Here's the drawing with two shaded views (mm, measured from the low corner). I have some questions. A direction names the side the tool comes from. Round coordinates to 2 decimals unless told otherwise and drop trailing zeros. Loops run counter-clockwise (first coordinate to the right, second up) from the corner with the lowest first, then second, coordinate; pieces in that order, holes last.
(1) If I drill on line 1 along Z through (x, y) = (16, 16); line 2 along X through (y, z) = (17.5, 56); line 3 along Z through (x, y) = (104, 17.75), over which ranges is the centre line in solid material (lowest first)?
(2) I want a section at C-C on z = 72. Write out the boundary of the cut face in (x, y).
(3) I want a section at A-A on y = 8. Write out the boundary of the cut face in (x, z) (1 decimal), plus the area to 3 significant figures.
(4) Will these pins go through, and if not, where does the flat tip stop? pin 1 Ø4 at (x, y) = (58, 11) entering from +Z; pin 2 Ø0.9 at (x, y) = (81.5, 17) entering from +Z; pin 3 Ø3 at (x, y) = (128, 16) entering from +Z.
(5) I want a section at B-B on x = 113. Write out the boundary of the cut face in (y, z).
(6) Which directions (+Z, -Z, +X, -X, +Y, -Y) give clear straight access to the entire face, cutting with the end or side of a thin tool? Please do the marked faces 1, 2 and 3.
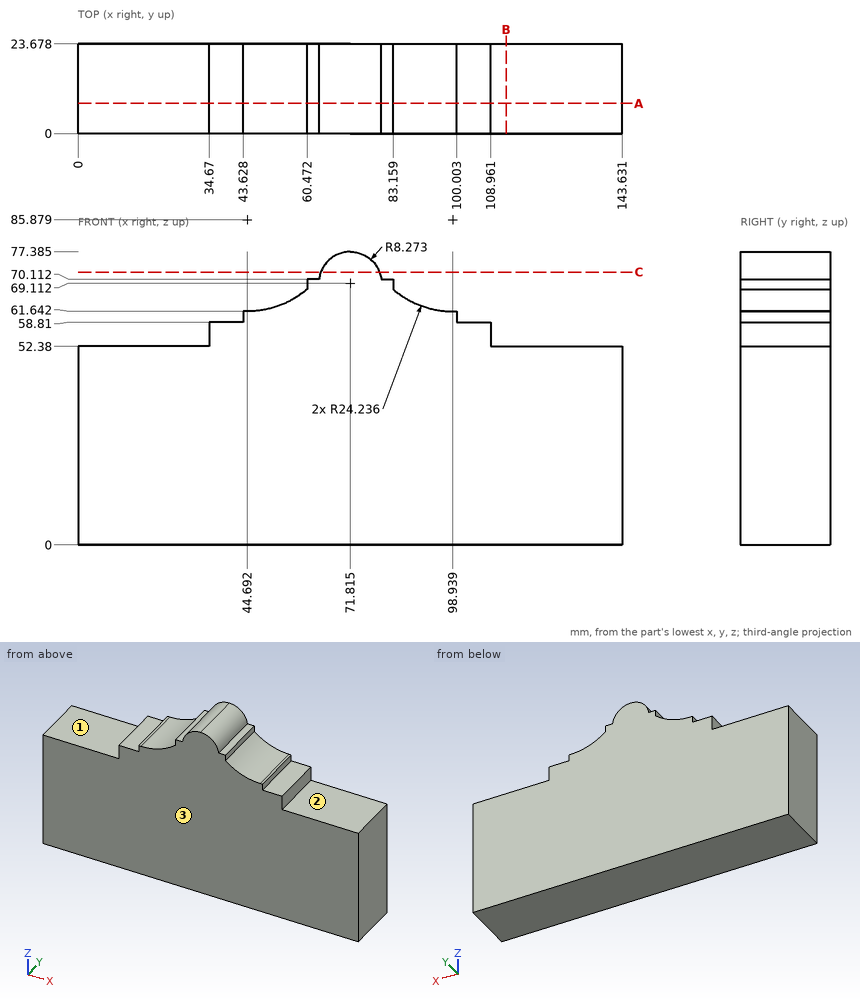
Filled sheet:
1. line 1: z = 0 to 52.38
1. line 2: x = 34.67 to 108.96
1. line 3: z = 0 to 58.81
2. outline: (64.06, 0) - (79.57, 0) - (79.57, 23.68) - (64.06, 23.68) - close
3. outline: (0, 0) - (143.6, 0) - (143.6, 52.4) - (109, 52.4) - (109, 58.8) - (100, 58.8) - (100, 61.6) - (98.9, 61.6) arc R24.2 cw to (83.2, 67.5) - (83.2, 70.1) - (80, 70.1) arc R8.3 ccw to (63.6, 70.1) - (60.5, 70.1) - (60.5, 67.5) arc R24.2 cw to (44.7, 61.6) - (43.6, 61.6) - (43.6, 58.8) - (34.7, 58.8) - (34.7, 52.4) - (0, 52.4) - close
3. area: 8,500 mm2
4. pin 1: stops at z = 67.09
4. pin 2: stops at z = 70.11
4. pin 3: stops at z = 52.38
5. outline: (0, 0) - (23.68, 0) - (23.68, 52.38) - (0, 52.38) - close
6. face 1: +Z, -X, +Y, -Y
6. face 2: +Z, +X, +Y, -Y
6. face 3: +Z, -Z, +X, -X, -Y
